Autodesk Inventor part; units mm, degrees
ref_plane "YZ Plane" through (0, 0, 0) normal (1, 0, 0) x (0, 1, 0)
ref_plane "XZ Plane" through (0, 0, 0) normal (0, 1, 0) x (-1, 0, 0)
ref_plane "XY Plane" through (0, 0, 0) normal (0, 0, 1) x (1, 0, 0)
sketch "Sketch1" plane through (0, 0, 0) normal (1, 0, 0) x (0, 1, 0)
  line L0 (-30, 21) -> (30, 21)
  line L1 (30, 21) -> (30, -21)
  line L2 (30, -21) -> (-30, -21)
  line L3 (-30, -21) -> (-30, 21)
  line L4 (-30, 21) -> (30, -21) construction
  line L5 (30, 21) -> (-30, -21) construction
  point P0 (0, 0)
  dimension "d0" = 60
  dimension "d1" = 42
extrude "Extrusion1" add sketch "Sketch1" along normal blind 2
chamfer "Chamfer1" distance 4 angle 45 4 edges at (1, -30, 21) (1, -30, -21) (1, 30, -21) (1, 30, 21)
sketch "Sketch2" plane through (2, 0, 0) normal (1, 0, 0) x (0, 0, -1)
  circle A0 centre (0, 0) radius 1
  dimension "d7" = 2
extrude "Extrusion2" cut sketch "Sketch2" against normal blind 2
properties part number "card"
Build history of the part. All positions in model axes, mm. Round coordinates to 2 decimals unless told otherwise and drop trailing zeros. Order: outer loops, then holes, each group sorted by start corner. A loop starts at its lowest first (then second) coordinate and runs counter-clockwise, first axis right, second up. Notation, with made-up numbers: M 20.25,14 L 47.25,14 A25 ccw 47.25,39 Z; hole C 82,80.25 d6. An arc over 180 degrees is marked long. Use CSV: the item, a comma, the result in double quotes. Start each with the question number.
(1) Cut at B-B on z = 0. List the corners of the cut face in (x, y).
(2) Cut at A-A on y = 0. List the corners of the cut face in (x, z).
(3) Mould opens along Y. For faces 1 (the face through (1, 28, 19)), 2 (the face through (1, -1, 0)), 3 (the face through (1, -28, 19)), 4 (the face through (1, 0, -21)) say: +Y half, -Y half, draft (parallel to the pull), parting line (faces both ways), or undercut.
(4) Drill centre lines: probe 1 along Y at (x, z) = (1, 0); probe 2 along Z at (x, y) = (0.9, -0.5); probe 3 along Y at (x, z) = (0.35, -0.5). Where is each one in solid material? Low to high.
Findings:
1,outline,"M 0,-30 L 2,-30 L 2,-1 L 0,-1 Z; M 0,1 L 2,1 L 2,30 L 0,30 Z"
2,outline,"M 0,-21 L 2,-21 L 2,-1 L 0,-1 Z; M 0,1 L 2,1 L 2,21 L 0,21 Z"
3,face 1,"+Y half"
3,face 2,"undercut"
3,face 3,"-Y half"
3,face 4,"draft"
4,probe 1,"y = -30 to -1, 1 to 30"
4,probe 2,"z = -21 to -0.87, 0.87 to 21"
4,probe 3,"y = -30 to -0.87, 0.87 to 30"
